Verification items for the finished model (mm, model axes). Face numbers are marked on the shaded views. Round coordinates to 2 decimals unless told otherwise and drop trailing zeros. Loops run counter-clockwise (first coordinate to the right, second up) from the corner with the lowest first, then second, coordinate; pieces in that order, holes last. Notation, with made-up numbers: (32, 79) - (56, 79) arc R19 ccw to (56, 90) - close; hole circle Ø5 at (-19.75, 79.25). An arc over 180 degrees is marked (long way). Use a Markdown table: item, result. Add a question column.
```python
from build123d import *

# Parameters (mm, degrees)
BOSS_EXTRU_1_DEPTH      = 2
CONG_1_R                = 10
CONG_3_R                = 4
CONG_4_R                = 1
BOSS_EXTRU_2_DEPTH      = 7
ENL_V_START             = -1
ENL_V_MAT_EXTRU_1_DEPTH = 1
ESQUISSE6_W             = 33
ESQUISSE6_H             = 3
BOSS_EXTRU_3_DEPTH      = 10


with BuildPart() as part:
    # Esquisse1 → Boss.-Extru.1 (new body)
    with BuildSketch(Plane(origin=(0, 0, 0), x_dir=(1, 0, 0), z_dir=(0, 1, 0))):
        Polygon((-70.5, 42.5), (-47.5, 42.5), (18, 42.5), (35, 42.5), (35, -15), (70.5, -15), (70.5, -42.5), (17.75, -42.5), (17.75, 4.5), (-47.75, 4.5), (-47.75, -42.5), (-70.5, -42.5), align=None)
    extrude(amount=BOSS_EXTRU_1_DEPTH)

    # Congé1
    cong_1_edges = [part.edges().sort_by_distance(p)[0] for p in [
        (35, 1, 15),
    ]]
    fillet(cong_1_edges, radius=CONG_1_R)

    # Congé3
    cong_3_edges = [part.edges().sort_by_distance(p)[0] for p in [
        (-70.5, 1, -42.5),
        (70.5, 1, 42.5),
        (-70.5, 1, 42.5),
    ]]
    fillet(cong_3_edges, radius=CONG_3_R)

    # Congé4
    cong_4_edges = [part.edges().sort_by_distance(p)[0] for p in [
        (17.75, 1, -4.5),
        (-47.75, 1, -4.5),
    ]]
    fillet(cong_4_edges, radius=CONG_4_R)

    # Esquisse3 → Boss.-Extru.2 (add)
    with BuildSketch(Plane(origin=(0, 2, 0), x_dir=(1, 0, 0), z_dir=(0, 1, 0))):
        with BuildLine():
            Line((-68.45, 38.5), (-68.45, -38.5))
            ThreePointArc((-68.45, -38.5), (-67.878858223, -39.878858223), (-66.5, -40.45))
            Line((-66.5, -40.45), (-47.75, -40.45))
            Line((-47.75, -40.45), (-47.75, -38.45))
            Line((-47.75, -38.45), (-66.5, -38.5))
            Line((-66.5, -38.5), (-66.5, 38.5))
            Line((-66.5, 38.5), (32.95, 38.5))
            Line((32.95, 38.5), (32.95, -5))
            ThreePointArc((32.95, -5), (36.479363287, -13.520636713), (45, -17.05))
            Line((45, -17.05), (66.5, -17.05))
            Line((66.5, -17.05), (66.5, -38.5))
            Line((66.5, -38.5), (17.75, -38.5))
            Line((17.75, -38.5), (17.75, -40.45))
            Line((17.75, -40.45), (66.5, -40.45))
            ThreePointArc((66.5, -40.45), (67.878858223, -39.878858223), (68.45, -38.5))
            Line((68.45, -38.5), (68.45, -15))
            Line((68.45, -15), (45, -15))
            ThreePointArc((45, -15), (37.928932188, -12.071067812), (35, -5))
            Line((35, -5), (35, 40.45))
            Line((35, 40.45), (-66.5, 40.45))
            ThreePointArc((-66.5, 40.45), (-67.878858223, 39.878858223), (-68.45, 38.5))
        make_face()
    extrude(amount=-BOSS_EXTRU_2_DEPTH)

    # Esquisse5 → Enlèv. mat.-Extru.1 (cut)
    with BuildSketch(Plane.XZ.offset(5).offset(ENL_V_START)):
        with BuildLine():
            Line((66.5, 40.45), (33.5, 40.45))
            Line((33.5, 40.45), (33.5, 38.5))
            Line((33.5, 38.5), (66.5, 38.5))
            Line((66.5, 38.5), (66.5, 24.5))
            Line((66.5, 24.5), (68.45, 24.5))
            Line((68.45, 24.5), (68.45, 38.5))
            ThreePointArc((68.45, 38.5), (67.878858223, 39.878858223), (66.5, 40.45))
        make_face()
    extrude(amount=ENL_V_MAT_EXTRU_1_DEPTH, mode=Mode.SUBTRACT)

    # Esquisse6 → Boss.-Extru.3 (add)
    with BuildSketch(Plane.XZ):
        with Locations((50, 24.5)):
            Rectangle(ESQUISSE6_W, ESQUISSE6_H)
    extrude(amount=BOSS_EXTRU_3_DEPTH)


solid = part.part
```
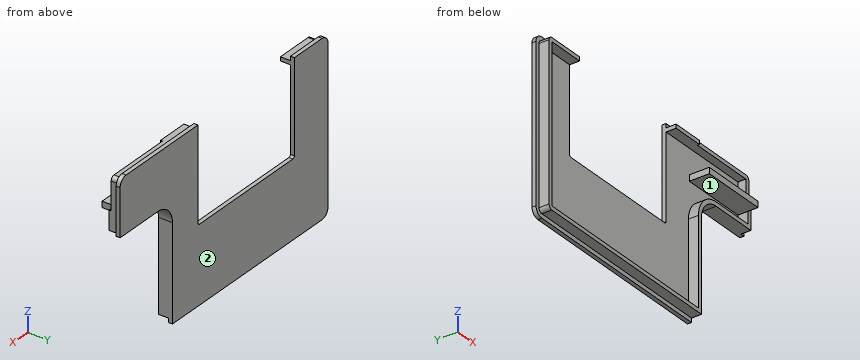
Q1. Section check A-A on x = 59.5. Record the cut outline in (y, z).
Q2. Section check B-B on y = -1.5. Record the cut outline in (x, z), plus the area to 3 significant figures.
Q3. Section check D-D on z = -9. Record the cut outline in (x, y), plus the area to 3 significant figures.
Q4. Section check C-C on z = 10.5. Record the cut outline in (x, y), plus the area to 3 significant figures.
Q5. Thickness scan on line 1 along Z through (x, y) = (60, -1.5); line 2 along X through (y, z) = (-0.75, 33); line 3 along Z through (x, y) = (59, -4.75). Record the ranges inside material, lowest first.
Q6. Release check for a two-part mould opening along Z. For the marked faces 1 and 2 record: +Z half, -Z half, draft (parallel to the pull), parting line (faces both ways), or undercut.
Q7. Go/stop test with flat-tipped pins: pin 1 Ø4 at (x, z) = (16.5, 28.5) entering from -Y; pin 2 Ø0.9 at (y, z) = (-6.5, 25) entering from -X; pin 3 Ø2.5 at (y, z) = (-1.5, -11) entering from -X. Record where each tip stops, or that it passes through.
Determined:
| question | item | result |
|---|---|---|
| 1 | outline | (-10, 23) - (0, 23) - (0, 17.05) - (-5, 17.05) - (-5, 15) - (2, 15) - (2, 42.5) - (0, 42.5) - (0, 40.45) - (-4, 40.45) - (-4, 38.5) - (0, 38.5) - (0, 26) - (-10, 26) - close |
| 2 | outline | (-68.45, -38.5) arc R1.95 ccw to (-66.5, -40.45) - (35, -40.45) - (35, 5) arc R10 cw to (45, 15) - (68.45, 15) - (68.45, 38.5) arc R1.95 ccw to (66.5, 40.45) - (17.75, 40.45) - (17.75, 38.5) - (66.5, 38.5) - (66.5, 26) - (33.5, 26) - (33.5, 23) - (66.5, 23) - (66.5, 17.05) - (45, 17.05) arc R12.05 ccw to (32.95, 5) - (32.95, -38.5) - (-66.5, -38.5) - (-66.5, 38.5) - (-47.75, 38.45) - (-47.75, 40.45) - (-66.5, 40.45) arc R1.95 ccw to (-68.45, 38.5) - close |
| 2 | area | 803 mm² |
| 3 | outline | (-70.5, 0) - (-68.45, 0) - (-68.45, -5) - (-66.5, -5) - (-66.5, 0) - (32.95, 0) - (32.95, -5) - (35, -5) - (35, 2) - (-70.5, 2) - close |
| 3 | area | 231 mm² |
| 4 | outline | (-70.5, 0) - (-68.45, 0) - (-68.45, -5) - (-66.5, -5) - (-66.5, 0) - (-47.75, 0) - (-47.75, 2) - (-70.5, 2) - close; (17.75, 0) - (34.28, 0) - (34.28, -5) - (36.65, -5) - (36.65, 2) - (17.75, 2) - close |
| 4 | area | 105 mm² |
| 5 | line 1 | z = 15 to 17.05, 23 to 26, 38.5 to 40.45 |
| 5 | line 2 | x = -68.45 to -66.5, 66.5 to 68.45 |
| 5 | line 3 | z = 15 to 17.05, 23 to 26 |
| 6 | face 1 | undercut |
| 6 | face 2 | draft |
| 7 | pin 1 | stops at y = 0 |
| 7 | pin 2 | stops at x = 33.5 |
| 7 | pin 3 | stops at x = -68.45 |
